from build123d import *

# Parameters (mm, degrees)
F0_W     = 81.28
F0_H     = 50.8
F1_DEPTH = 3
F2_W     = 3.6068
F2_H     = 5.0038
F3_DEPTH = 5.588
F2_W_2   = 3.302
F2_H_2   = 4.4958
F4_DEPTH = 8.9916
F6_DEPTH = 3.5052
F9_DEPTH = 3.5052


with BuildPart() as f1:
    # F0 (on Front) → F1 (new body)
    with BuildSketch(Plane.XZ):
        Rectangle(F0_W, F0_H)
    extrude(amount=F1_DEPTH)

    # F2 (on face) → F3 (join)
    with BuildSketch(Plane(origin=(0, 0, 0), x_dir=(-1, 0, 0), z_dir=(0, 1, 0))):
        with Locations((38.8366, 22.8981)):
            Rectangle(F2_W, F2_H)
        with Locations((-38.8366, 22.8981)):
            Rectangle(F2_W, F2_H)
        with Locations((-15.0818, 22.8981)):
            Rectangle(F2_W, F2_H)
        with Locations((15.0818, 22.8981)):
            Rectangle(F2_W, F2_H)
    extrude(amount=F3_DEPTH)

    # F2 (on face) → F4 (join)
    with BuildSketch(Plane(origin=(0, 0, 0), x_dir=(-1, 0, 0), z_dir=(0, 1, 0))):
        with Locations((-38.989, -1.8415)):
            Rectangle(F2_W_2, F2_H_2)
        with Locations((38.989, -1.8415)):
            Rectangle(F2_W_2, F2_H_2)
    extrude(amount=F4_DEPTH)

    # F5 (on face) → F6 (join)
    with BuildSketch(Plane(origin=(-40.64, 0, 0), x_dir=(0, -1, 0), z_dir=(-1, 0, 0))):
        with BuildLine():
            Line((-10.3632, 30.4038), (-10.3632, 25.4))
            ThreePointArc((-10.3632, 25.4), (-9.046343, 21.876274), (-5.588, 20.3962))
            Line((-5.588, 20.3962), (-5.588, 25.4))
            ThreePointArc((-5.588, 25.4), (-8.070259, 27.349257), (-8.8646, 30.4038))
            Line((-8.8646, 30.4038), (-10.3632, 30.4038))
        make_face()
    extrude(amount=-F6_DEPTH)

    # F7: F1 across plane


with BuildPart() as f1_1:
    add(f1.part)
    add(f1.part.mirror(Plane.YZ))

    # F8 (on face) → F9 (join)
    with BuildSketch(Plane(origin=(-16.8852, 0, 0), x_dir=(0, -1, 0), z_dir=(-1, 0, 0))):
        with BuildLine():
            Line((-8.5852, 30.4038), (-8.5852, 25.4))
            ThreePointArc((-8.5852, 25.4), (-7.77858, 22.483614), (-5.588, 20.3962))
            Line((-5.588, 20.3962), (-5.588, 25.4))
            ThreePointArc((-5.588, 25.4), (-6.915574, 27.728711), (-7.0866, 30.4038))
            Line((-7.0866, 30.4038), (-8.5852, 30.4038))
        make_face()
    extrude(amount=-F9_DEPTH)

    # F10: F1 across plane


with BuildPart() as f1_2:
    add(f1_1.part)
    add(f1_1.part.mirror(Plane.YZ))


solid = f1_2.part
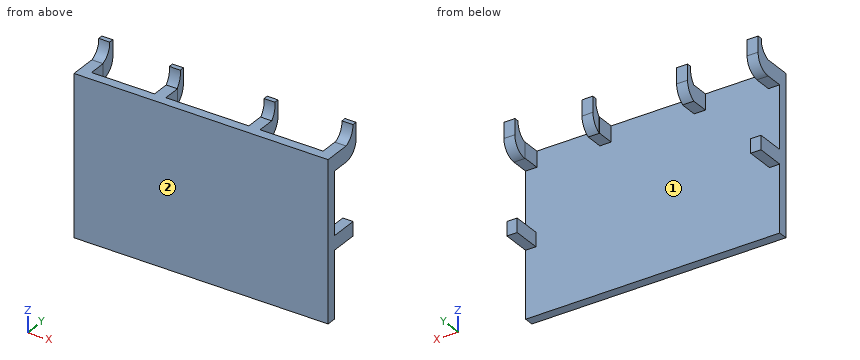
The model under review builds one solid part; all positions refer to its coordinate system, in mm. Face numbers are marked on the shaded views. Give positions to 0.01 mm unless a question says otherwise; leave off trailing zeros. Order: outer loops, then holes, each group sorted by start corner. A loop starts at its lowest first (then second) coordinate and runs counter-clockwise, first axis right, second up. Notation, with made-up numbers: M 42.5,26 L 94.5,26 A23 cw 94.5,53 Z; hole C 2,2 d7. An arc over 180 degrees is marked long. Answer in a Markdown table with one row per item. Add a question column.
1. Add section D-D on z = -19. State the section outline as (x, y) points, plus the area to 3 significant figures.
2. Add section C-C on x = 22. State the section outline as (y, z) points.
3. For pin 1 Ø4 at (x, z) = (38.5, 27.5) entering from +Y; pin 2 Ø2.5 at (x, z) = (39.5, -3) entering from +Y; pin 3 Ø1.1 at (x, z) = (-14.5, 28) entering from +Y, all flat-tipped, find the tip position at first contact; note any pin that passes through.
4. Mouldability with a two-part tool opening along X and no side actions: class the marked faces 1 and 2 as released by +X, released by -X, zero draft, split by the parting line, or undercut.
5. Add section B-B on z = -2. State the section outline as (x, y) points, plus the area to 3 significant figures.
6. Add section A-A on y = 1.75. State the section outline as (x, z) points.
7. To check wall thickness, follow line 1 along X through (y, z) = (3.5, 25); line 2 along X through (y, z) = (5.75, 25.5); line 3 along X through (y, z) = (1.25, -3.5). State the ranges of each line that lie inside material, in increasing order.
The answers:
| question | item | result |
|---|---|---|
| 1 | outline | M -40.64,-3 L 40.64,-3 L 40.64,0 L -40.64,0 Z |
| 1 | area | 244 mm2 |
| 2 | outline | M -3,-25.4 L 0,-25.4 L 0,25.4 L -3,25.4 Z |
| 3 | pin 1 | y = 10.36 |
| 3 | pin 2 | y = 8.99 |
| 3 | pin 3 | y = 8.59 |
| 4 | face 1 | undercut |
| 4 | face 2 | zero draft |
| 5 | outline | M -40.64,-3 L 40.64,-3 L 40.64,8.99 L 37.34,8.99 L 37.34,0 L -37.34,0 L -37.34,8.99 L -40.64,8.99 Z |
| 5 | area | 303 mm2 |
| 6 | outline | M -40.64,-4.09 L -37.34,-4.09 L -37.34,0.41 L -40.64,0.41 Z; M -40.64,20.4 L -37.03,20.4 L -37.03,25.4 L -40.64,25.4 Z; M -16.89,20.4 L -13.28,20.4 L -13.28,25.4 L -16.89,25.4 Z; M 13.28,20.4 L 16.89,20.4 L 16.89,25.4 L 13.28,25.4 Z; M 37.03,20.4 L 40.64,20.4 L 40.64,25.4 L 37.03,25.4 Z; M 37.34,-4.09 L 40.64,-4.09 L 40.64,0.41 L 37.34,0.41 Z |
| 7 | line 1 | -40.64 to -37.03, -16.89 to -13.28, 13.28 to 16.89, 37.03 to 40.64 |
| 7 | line 2 | -16.89 to -13.38, 13.38 to 16.89 |
| 7 | line 3 | -40.64 to -37.34, 37.34 to 40.64 |
